Check sheet for the modelled part. Datum: model origin and axes. Units: mm. Round coordinates to 2 decimals unless told otherwise and drop trailing zeros. Write each loop counter-clockwise with the first axis right and the second up, starting at its lowest first coordinate (ties: lowest second). Pieces come first, ordered by that corner, then holes. Notation, with made-up numbers: M 69.5,66 L 74.5,66 A22 cw 74.5,102 Z; hole C -28.75,33.25 d2. An arc over 180 degrees is marked long. Answer in a Markdown table with one row per item.
```python
from build123d import *

# Parameters (mm, degrees)
F4_DEPTH = 25
F6_DEPTH = 25


# Not quite as in the source:
# - the dataset's text gives a spline's control points without its knots; the knots are read off the source's solid


with BuildPart() as f1:
    # F0 (on Front) → F1 (revolve)
    with BuildSketch(Plane.XZ):
        with BuildLine():
            Line((20.2840724203, -27.343348276), (23.0495763149, -27.3330021896))
            Line((23.0495763149, -27.3330021896), (23.0495763149, 24.1761978883))
            add(Edge.make_bspline(
                [(23.0495763149, 24.1761978883), (22.8941435237, 26.0308608144), (23.9395420726, 29.003648868), (14.0261189654, 33.6296849109), (8.4189805979, 34.9379997258)],
                knots=[0, 0, 0, 0, 0.3260886129, 0.8771804513, 0.8771804513, 0.8771804513, 0.8771804513], degree=3))
            add(Edge.make_bspline(
                [(8.4189805979, 34.9379997258), (8.1849872822, 34.992597437), (7.9520754508, 35.0444122094), (7.7206045906, 35.0932804837)],
                knots=[0.8771804513, 0.8771804513, 0.8771804513, 0.8771804513, 0.9001782441, 0.9001782441, 0.9001782441, 0.9001782441], degree=3))
            add(Edge.make_bspline(
                [(7.7206045906, 35.0932804837), (6.7159069707, 35.3053928798), (5.7383570717, 35.4619936087), (4.8173516989, 35.5497077107)],
                knots=[0.9001782441, 0.9001782441, 0.9001782441, 0.9001782441, 1, 1, 1, 1], degree=3))
            Line((4.8173516989, 35.5497077107), (0, 35.5497077107))
            Line((0, 35.5497077107), (0, 34.6961133182))
            Line((0, 34.6961133182), (4.8552267253, 34.6961133182))
            add(Edge.make_bspline(
                [(22.3495763149, 23.4555121765), (22.1897726726, 25.3623291907), (23.6752847702, 29.0289436305), (10.9884647614, 34.112000041), (4.8552267253, 34.6961133182)],
                knots=[0, 0, 0, 0, 0.3352583947, 1, 1, 1, 1], degree=3))
            Line((22.3495763149, 23.4555121765), (22.3495763149, -26.6947299242))
            Line((22.3495763149, -26.6947299242), (0, -26.6947299242))
            Line((0, -26.6947299242), (0, -27.4192334573))
            Line((0, -27.4192334573), (8.9649282769, -27.3856945706))
            Line((8.9649282769, -27.3856945706), (9.7, -27.3829445779))
            Line((9.7, -27.3829445779), (18.8340822147, -27.3487728656))
            Line((18.8340822147, -27.3487728656), (20.2840724203, -27.343348276))
        make_face()
    revolve(axis=Axis((0, 0, -7.0726890117), (0, 0, -1)))

    # F0 (on Front) → F2 (revolve)
    with BuildSketch(Plane.XZ):
        with BuildLine():
            add(Edge.make_bspline(
                [(23.0495763149, -60.2150011641), (22.8941435237, -58.3603382379), (23.8898585914, -55.5288345389), (14.9436544002, -51.1974927604), (9.7, -49.7765717533)],
                knots=[0, 0, 0, 0, 0.3260886129, 0.8354916825, 0.8354916825, 0.8354916825, 0.8354916825], degree=3))
            add(Edge.make_bspline(
                [(9.7, -49.7765717533), (9.4543795426, -49.7100137308), (9.2092217969, -49.6461323577), (8.9649282769, -49.5851103148)],
                knots=[0.8354916825, 0.8354916825, 0.8354916825, 0.8354916825, 0.8593528689, 0.8593528689, 0.8593528689, 0.8593528689], degree=3))
            add(Edge.make_bspline(
                [(8.9649282769, -49.5851103148), (7.5249670698, -49.2254226142), (6.1150323727, -48.9650789974), (4.8173516989, -48.8414913416)],
                knots=[0.8593528689, 0.8593528689, 0.8593528689, 0.8593528689, 1, 1, 1, 1], degree=3))
            Line((4.8173516989, -48.8414913416), (0, -48.8414913416))
            Line((0, -48.8414913416), (0, -49.6950857341))
            Line((0, -49.6950857341), (4.8552267253, -49.6950857341))
            add(Edge.make_bspline(
                [(22.3156850975, -60.2261610329), (22.2921596802, -58.7073440576), (23.1236631734, -55.1412446649), (10.9884647614, -50.2791990114), (4.8552267253, -49.6950857341)],
                knots=[0.0434798946, 0.0434798946, 0.0434798946, 0.0434798946, 0.3352583947, 1, 1, 1, 1], degree=3))
            add(Edge.make_bspline(
                [(22.3495763149, -60.9356868758), (22.3288512693, -60.6883904498), (22.3191907796, -60.4524902586), (22.3156850975, -60.2261610329)],
                knots=[0, 0, 0, 0, 0.0434798946, 0.0434798946, 0.0434798946, 0.0434798946], degree=3))
            Line((22.3495763149, -60.9356868758), (23.0495763149, -60.9422326088))
            Line((23.0495763149, -60.9422326088), (23.0495763149, -60.2150011641))
        make_face()
        with BuildLine():
            Line((9.7, -49.5851103148), (9.7, -27.3829445779))
            Line((9.7, -27.3829445779), (8.9649282769, -27.3856945706))
            Line((8.9649282769, -27.3856945706), (8.9649282769, -28.0694384128))
            Line((8.9649282769, -28.0694384128), (8.9649282769, -49.5851103148))
            add(Edge.make_bspline(
                [(9.7, -49.7765717533), (9.4543795426, -49.7100137308), (9.2092217969, -49.6461323577), (8.9649282769, -49.5851103148)],
                knots=[0.8354916825, 0.8354916825, 0.8354916825, 0.8354916825, 0.8593528689, 0.8593528689, 0.8593528689, 0.8593528689], degree=3))
            Line((9.7, -49.7765717533), (9.7, -49.5851103148))
        make_face()
        with BuildLine():
            Line((0, -60.9356868758), (22.3495763149, -60.9356868758))
            add(Edge.make_bspline(
                [(22.3495763149, -60.9356868758), (22.3288512693, -60.6883904498), (22.3191907796, -60.4524902586), (22.3156850975, -60.2261610329)],
                knots=[0, 0, 0, 0, 0.0434798946, 0.0434798946, 0.0434798946, 0.0434798946], degree=3))
            Line((22.3156850975, -60.2261610329), (0, -60.2261610329))
            Line((0, -60.2261610329), (0, -60.9356868758))
        make_face()
        Polygon((8.9649282769, -28.0694384128), (8.9649282769, -27.3856945706), (0, -27.4192334573), (0, -28.0694384128), align=None)
    revolve(axis=Axis((0, 0, -7.0726890117), (0, 0, -1)))

    # F3 (on Right) → F4 (cut, symmetric)
    with BuildSketch(Plane.YZ):
        with BuildLine():
            Line((-10.9680155292, -4.0999995545), (-0.0928910449, -4.0999995545))
            Line((-0.0928910449, -4.0999995545), (10.7822334394, -4.0999995545))
            Line((10.7822334394, -4.0999995545), (10.7822334394, 1.6936261673))
            add(Edge.make_bspline(
                [(10.7822334394, 1.6936261673), (10.8915483579, 10.6573491357), (8.377331309, 12.5156822614), (-0.0928910449, 14.0460734256)],
                knots=[0, 0, 0, 0, 16.4575601417, 16.4575601417, 16.4575601417, 16.4575601417], degree=3))
            add(Edge.make_bspline(
                [(-10.9680155292, 1.6936261673), (-11.0773304477, 10.6573491357), (-8.5631133988, 12.5156822614), (-0.0928910449, 14.0460734256)],
                knots=[0, 0, 0, 0, 16.4575601417, 16.4575601417, 16.4575601417, 16.4575601417], degree=3))
            Line((-10.9680155292, 1.6936261673), (-10.9680155292, -4.0999995545))
        make_face()
    extrude(amount=F4_DEPTH, both=True, mode=Mode.SUBTRACT)

    # F5 (on Front) → F6 (cut, symmetric)
    with BuildSketch(Plane.XZ):
        with BuildLine():
            Line((-10.8819976449, -3.9999997243), (-0.0068731606, -3.9999997243))
            Line((-0.0068731606, -3.9999997243), (10.8682513237, -3.9999997243))
            Line((10.8682513237, -3.9999997243), (10.8682513237, 1.7936259974))
            add(Edge.make_bspline(
                [(10.8682513237, 1.7936259974), (10.9775662422, 10.7573489659), (8.4633491933, 12.6156820916), (-0.0068731606, 14.1460732557)],
                knots=[0, 0, 0, 0, 16.4575601417, 16.4575601417, 16.4575601417, 16.4575601417], degree=3))
            add(Edge.make_bspline(
                [(-10.8819976449, 1.7936259974), (-10.9913125634, 10.7573489659), (-8.4770955145, 12.6156820916), (-0.0068731606, 14.1460732557)],
                knots=[0, 0, 0, 0, 16.4575601417, 16.4575601417, 16.4575601417, 16.4575601417], degree=3))
            Line((-10.8819976449, 1.7936259974), (-10.8819976449, -3.9999997243))
        make_face()
    extrude(amount=F6_DEPTH, both=True, mode=Mode.SUBTRACT)

    # F0 (on Front) → F7 (revolve)
    with BuildSketch(Plane.XZ):
        with BuildLine():
            add(Edge.make_bspline(
                [(8.4189805979, 34.9379997258), (8.1849872822, 34.992597437), (7.9520754508, 35.0444122094), (7.7206045906, 35.0932804837)],
                knots=[0.8771804513, 0.8771804513, 0.8771804513, 0.8771804513, 0.9001782441, 0.9001782441, 0.9001782441, 0.9001782441], degree=3))
            Line((8.4189805979, 34.9379997258), (8.865498937, 76.6738313739))
            Line((8.865498937, 76.6738313739), (23.0495763148, 76.6738313739))
            Line((23.0495763148, 76.6738313739), (23.0495763148, 78.7230981444))
            add(Edge.make_bspline(
                [(23.0495763148, 78.7230981444), (23.0495763148, 80.6078122564), (23.9507031304, 83.9578134153), (11.2077367667, 90.5497077107), (5, 90.5497077107)],
                knots=[0, 0, 0, 0, 0.3302146344, 1, 1, 1, 1], degree=3))
            Line((5, 90.5497077107), (0, 90.5497077107))
            Line((0, 90.5497077107), (0, 89.8497104645))
            Line((0, 89.8497104645), (5, 89.8497104645))
            add(Edge.make_bspline(
                [(22.3495790686, 78.7230981444), (22.3495790686, 79.0937647853), (22.3716877562, 79.7678791576), (22.3933148354, 80.6007538754), (22.3399061529, 81.2821155275), (22.1725915882, 81.8776125403), (21.8790408964, 82.4045882825), (21.4922195357, 82.886710278), (20.9908563885, 83.4132154485), (20.1707115884, 84.1274223788), (18.9256521099, 85.0269281278), (17.4668159276, 85.9325369699), (15.2961373534, 87.1052139435), (12.269445396, 88.4292040949), (8.4841313235, 89.5564062965), (6.0965880095, 89.8497104645), (5, 89.8497104645)],
                knots=[0, 0, 0, 0, 0.0625, 0.125, 0.1875, 0.25, 0.3125, 0.34375, 0.375, 0.4375, 0.5, 0.5625, 0.625, 0.75, 0.875, 1, 1, 1, 1], degree=3))
            Line((22.3495790686, 78.7230981444), (22.3495790686, 77.3738286202))
            Line((22.3495790686, 77.3738286202), (8.1729506775, 77.3738286202))
            Line((8.1729506775, 77.3738286202), (7.7206045906, 35.0932804837))
        make_face()
    revolve(axis=Axis((0, 0, 62.5293496996), (0, 0, -1)))


solid = f1.part
```
1. Section check C-C, the plane z = -38. Record the cut outline in (x, y), and give its area (3 significant figures).
Found:
| item | result |
|---|---|
| outline | C 0,0 d19.4; hole C 0,0 d17.93 |
| area | 43.1 mm2 |
2. Section check A-A, the plane x = -14.5. Count the separate pieces of the cut face and the enclosed holes in it, and give its area (3 significant figures).
Found:
| item | result |
|---|---|
| separate pieces | 3 |
| enclosed holes | 3 |
| area | 272 mm2 |
3. Go/stop test with flat-tipped pins: pin 1 (8 mm diameter, centred on x = 0, y = -1.5, fed in from -Z); pin 2 (3 mm diameter, centred on x = -3.5, y = 13.5, fed in from +Z); pin 3 (8 mm diameter, centred on y = 10, z = -26, fed in from -X). Record where each tip stops, or that it passes through.
Found:
| item | result |
|---|---|
| pin 1 | stops at z = -60.94 |
| pin 2 | stops at z = 89.02 |
| pin 3 | stops at x = -22.25 |
4. Scan lines: L1, parallel to Y at x = 0.5, z = 23; L2, parallel to Z at x = 9.5, y = -1; L3, parallel to Z at x = -9.5, y = 16. Record each from-to range of solid material in increasing order.
Found:
| item | result |
|---|---|
| L1 | y = -23.04 to -22.34, 22.34 to 23.04 |
| L2 | z = -60.94 to -60.23, -50.55 to -26.69, 33.84 to 34.65, 76.67 to 77.37, 89.2 to 89.92 |
| L3 | z = -60.94 to -60.23, -54.1 to -53.31, -27.35 to -26.69, 30.29 to 31.08, 76.67 to 77.37, 85.21 to 86.04 |
5. Draft check along Z on faces 1 (the face through (9.252, -2.914, -38.423)), 2 (the face through (21.985, -6.923, -60.574)), 3 (the face through (0, 0, 90.55)). Enter one of: +Z half, -Z half, draft (parallel to the pull), parting line (faces both ways), or undercut.
Found:
| item | result |
|---|---|
| face 1 | undercut |
| face 2 | draft |
| face 3 | +Z half |
